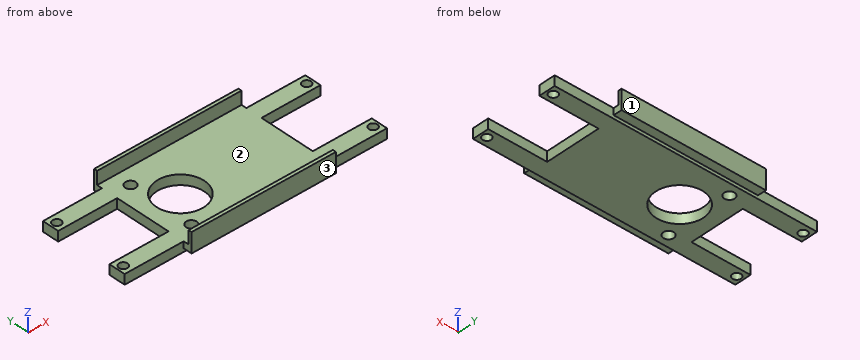
```python
from build123d import *

# Parameters (mm, degrees)
RESSALTO_EXTRUS_O1_DEPTH = 3
ESBO_O2_R                = 1.3
CORTE_EXTRUS_O1_DEPTH    = 3
ESBO_O3_W                = 2
ESBO_O3_H                = 16.9
RESSALTO_EXTRUS_O2_DEPTH = 3
ESBO_O4_R                = 7.25
CORTE_EXTRUS_O2_DEPTH    = 3
ESBO_O6_R                = 1.6
CORTE_EXTRUS_O3_DEPTH    = 3
ESBO_O7_W                = 44
ESBO_O7_H                = 2.6
RESSALTO_EXTRUS_O4_DEPTH = 2
ESBO_O8_W                = 44
ESBO_O8_H                = 1
RESSALTO_EXTRUS_O5_DEPTH = 4


with BuildPart() as part:
    # Esboço1 → Ressalto-extrusão1 (new body)
    with BuildSketch(Plane.XY):
        Polygon((-40, 0), (40, 0), (40, 5), (20, 5), (20, 21.9), (40, 21.9), (40, 26.9), (-40, 26.9), (-40, 21.9), (-20, 21.9), (-20, 5), (-40, 5), align=None)
    extrude(amount=RESSALTO_EXTRUS_O1_DEPTH)

    # Esboço2 → Corte-extrusão1 (cut)
    with BuildSketch(Plane.XY.offset(3)):
        with Locations((-38.1, 24.4)):
            Circle(ESBO_O2_R)
        with Locations((38.1, 24.4)):
            Circle(ESBO_O2_R)
        with Locations(Location((38.1, 2.5, 0), (0, 0, 180))):
            Circle(ESBO_O2_R)
        with Locations(Location((-38.1, 2.5, 0), (0, 0, 180))):
            Circle(ESBO_O2_R)
    extrude(amount=-CORTE_EXTRUS_O1_DEPTH, mode=Mode.SUBTRACT)

    # Esboço3 → Ressalto-extrusão2 (add)
    with BuildSketch(Plane.XY.offset(3)):
        with Locations((-21, 13.45)):
            Rectangle(ESBO_O3_W, ESBO_O3_H)
        with Locations((21, 13.45)):
            Rectangle(ESBO_O3_W, ESBO_O3_H)
    extrude(amount=-RESSALTO_EXTRUS_O2_DEPTH)

    # Esboço4 → Corte-extrusão2 (cut)
    with BuildSketch(Plane.XY.offset(3)):
        with Locations((-10.55, 13.45)):
            Circle(ESBO_O4_R)
    extrude(amount=-CORTE_EXTRUS_O2_DEPTH, mode=Mode.SUBTRACT)

    # Esboço6 → Corte-extrusão3 (cut)
    with BuildSketch(Plane.XY.offset(3)):
        with Locations((-16.47, 23.47)):
            Circle(ESBO_O6_R)
        with Locations(Location((-16.47, 3.43, 0), (0, 0, 180))):
            Circle(ESBO_O6_R)
    extrude(amount=-CORTE_EXTRUS_O3_DEPTH, mode=Mode.SUBTRACT)

    # Esboço7 → Ressalto-extrusão4 (add)
    with BuildSketch(Plane.XY.offset(3)):
        with Locations((0, 28.2)):
            Rectangle(ESBO_O7_W, ESBO_O7_H)
        with Locations((0, -1.3)):
            Rectangle(ESBO_O7_W, ESBO_O7_H)
    extrude(amount=-RESSALTO_EXTRUS_O4_DEPTH)

    # Esboço8 → Ressalto-extrusão5 (add)
    with BuildSketch(Plane.XY.offset(3)):
        with Locations((0, 29)):
            Rectangle(ESBO_O8_W, ESBO_O8_H)
        with Locations((0, -2.1)):
            Rectangle(ESBO_O8_W, ESBO_O8_H)
    extrude(amount=RESSALTO_EXTRUS_O5_DEPTH)


solid = part.part
```
Input: part model. Units: mm. Frame: model coordinates. Face numbers are marked on the shaded views. Give positions to 0.01 mm unless a question says otherwise; leave off trailing zeros. Order: outer loops, then holes, each group sorted by start corner. A loop starts at its lowest first (then second) coordinate and runs counter-clockwise, first axis right, second up. Notation, with made-up numbers: M 22,16 L 77,16 A10 cw 77,25 Z; hole C -7.75,56.25 d9. An arc over 180 degrees is marked long. Return JSON: item names as keys, results as strings.
1) Section query A-A on x = 26. Output: boundary loops of the cut face in (y, z).
Taken from the geometry:
{"outline": "M 0,0 L 5,0 L 5,3 L 0,3 Z; M 21.9,0 L 26.9,0 L 26.9,3 L 21.9,3 Z"}
2) Section query B-B on y = 13.45. Output: boundary loops of the cut face in (x, z).
Taken from the geometry:
{"outline": "M -22,0 L -17.8,0 L -17.8,3 L -22,3 Z; M -3.3,0 L 22,0 L 22,3 L -3.3,3 Z"}
3) Line query: L1, parallel to Y at x = 38.1, z = 1.1; L2, parallel to X at y = 24, z = 2.25; L3, parallel to X at y = 2.5, z = 1.7. Output: solid intervals per line, ascending. Write a range as [from, to].
Taken from the geometry:
{"L1": "y = [0, 1.2], [3.8, 5], [21.9, 23.1], [25.7, 26.9]", "L2": "x = [-40, -39.34], [-36.86, -17.98], [-14.96, 36.86], [39.34, 40]", "L3": "x = [-40, -39.4], [-36.8, -17.77], [-15.17, 36.8], [39.4, 40]"}
4) Section query C-C on x = -38.1. Output: boundary loops of the cut face in (y, z).
Taken from the geometry:
{"outline": "M 0,0 L 1.2,0 L 1.2,3 L 0,3 Z; M 3.8,0 L 5,0 L 5,3 L 3.8,3 Z; M 21.9,0 L 23.1,0 L 23.1,3 L 21.9,3 Z; M 25.7,0 L 26.9,0 L 26.9,3 L 25.7,3 Z"}
5) Contact query for flat-ended pins moving along their axis: pin 1 (2.5 mm diameter, centred on x = 35, z = 1.5, fed in from -Y); pin 2 (3 mm diameter, centred on x = -38.1, y = 2.5, fed in from +Z); pin 3 (3.5 mm diameter, centred on y = 12, z = 1, fed in from -X); pin 4 (3 mm diameter, centred on x = -16.47, y = 3.43, fed in from +Z). Output: stop coordinate, or through.
Taken from the geometry:
{"pin 1": "stops at y = 0", "pin 2": "stops at z = 3", "pin 3": "stops at x = -22", "pin 4": "passes through"}
6) Section query D-D on x = 16. Output: boundary loops of the cut face in (y, z), and give its area (3 significant figures).
Taken from the geometry:
{"outline": "M -2.6,1 L 0,1 L 0,0 L 26.9,0 L 26.9,1 L 29.5,1 L 29.5,7 L 28.5,7 L 28.5,3 L -1.6,3 L -1.6,7 L -2.6,7 Z", "area": "99.1 mm2"}
7) Mould query, pull axis Y, two halves, no side actions, for the marked faces 1, 2 and 3. Classes: released by +Y, released by -Y, zero draft, split by the parting line, or undercut.
Taken from the geometry:
{"face 1": "released by +Y", "face 2": "undercut", "face 3": "released by -Y"}
